from build123d import *

# Parameters (mm, degrees)
EXTRUDE_1_DEPTH     = 20
EXTRUDE_2_DEPTH     = 20
SKETCH_11_W         = 6.4
SKETCH_11_H         = 6.4
CUT_EXTRUDE_2_DEPTH = 13.1
SKETCH_4_R          = 1.6
CUT_EXTRUDE_1_DEPTH = 9.2


with BuildPart() as part:
    # 草图3 → 凸台-拉伸1 (new body)
    with BuildSketch(Plane.XY):
        Polygon((0, 0), (20, -12.790533612), (20, -72.995577455), (0, -72.995577455), align=None)
    extrude(amount=EXTRUDE_1_DEPTH)

    # 草图6 → 凸台-拉伸2 (add)
    with BuildSketch(Plane.XY.offset(20)):
        Polygon((0, -72.995577455), (-15, -72.995577455), (-15, -69.995577455), (0, 0), (0, -69.995577455), align=None)
    extrude(amount=-EXTRUDE_2_DEPTH)

    # 草图11 → 切除-拉伸2 (cut)
    with BuildSketch(Plane.XY.offset(20)):
        with Locations((-7.5, -66.995577455)):
            Rectangle(SKETCH_11_W, SKETCH_11_H)
        with Locations((10, -66.995577455)):
            Rectangle(SKETCH_11_W, SKETCH_11_H)
    extrude(amount=-CUT_EXTRUDE_2_DEPTH, mode=Mode.SUBTRACT)

    # 草图4 → 切除-拉伸1 (cut)
    with BuildSketch(Plane.XZ.offset(72.995577455)):
        with Locations(Location((10, 10, 0), (0, 0, 270))):
            Circle(SKETCH_4_R)
        with Locations(Location((-7.5, 10, 0), (0, 0, 270))):
            Circle(SKETCH_4_R)
    extrude(amount=-CUT_EXTRUDE_1_DEPTH, mode=Mode.SUBTRACT)


solid = part.part
Here's how the part is built. I have some questions about the finished solid (model axes, mm). A direction names the side the tool comes from. Give positions to 0.01 mm unless a question says otherwise; leave off trailing zeros. Loops run counter-clockwise (first coordinate to the right, second up) from the corner with the lowest first, then second, coordinate; pieces in that order, holes last. Notation, with made-up numbers: (88.5, -28.5) -> (96.5, -28.5) arc R20 ccw to (96.5, -8.5) -> close; hole circle Ø5 at (-17.5, -14.75). An arc over 180 degrees is marked (long way). Answer as a JSON object with one key per item and string values. Group by question number.
Item 1: Imagine slicing it at C-C on z = 10. Write out the boundary of the cut face in (x, y), then the cut area to 3 significant figures.
Item 2: I need wall thicknesses on L1, parallel to X at y = -71, z = 10; L2, parallel to Y at x = 9, z = 12.75; L3, parallel to Y at x = 7.5, z = 11.5. Which ranges of each line are inside material? Lowest first, please.
Item 3: On a 3-axis mill with a long thin cutter (end or side, diameter ignored), from which of +Z, -Z, +X, -X, +Y, -Y can I reach the whole of each face in a straight line? I mean faces 4 (the cylindrical face through (-8.47, -71.62, 11.27)), 5 (the flat face through (-4.3, -67, 14)), 6 (the flat face through (7, -44, 20)). Say none if no direction works.
Item 4: Will these pins go through, and if not, where does the flat tip stop? pin 1 (7 mm diameter, centred on x = 9.5, z = 11.5, fed in from +Y); pin 2 (1.9 mm diameter, centred on y = -65.5, z = 14, fed in from -X); pin 3 (3.5 mm diameter, centred on x = 10, z = 10, fed in from +Y).
Item 5: Thinking about a two-plate mould opening in Y: for faces 1 (the flat face through (3, -72.996, 10)), 2 (the flat face through (6.8, -67, 14)), 3 (the flat face through (-15, -72, 10)), which applies, pulls with the +Y half, pulls with the -Y half, needs draft (parallel to the pull), parting line crosses it, or undercut?
Item 6: Imagine slicing it at B-B on x = 10. Write out the boundary of the cut face in (y, z).
Item 7: Imagine slicing it at A-A on z = 15.25. Write out the boundary of the cut face in (x, y).
Item 8: Imagine slicing it at D-D on x = -7.5. Write out the boundary of the cut face in (y, z).
Answer list:
{
 "1": {"outline": "(-15, -73) -> (-9.1, -73) -> (-9.1, -70.2) -> (-10.7, -70.2) -> (-10.7, -63.8) -> (-4.3, -63.8) -> (-4.3, -70.2) -> (-5.9, -70.2) -> (-5.9, -73) -> (8.4, -73) -> (8.4, -70.2) -> (6.8, -70.2) -> (6.8, -63.8) -> (13.2, -63.8) -> (13.2, -70.2) -> (11.6, -70.2) -> (11.6, -73) -> (20, -73) -> (20, -12.79) -> (0, 0) -> (-15, -70) -> close", "area": "1,800 mm2"},
 "2": {"L1": "x = -15 to -9.1, -5.9 to 8.4, 11.6 to 20", "L2": "y = -73 to -70.2, -63.8 to -5.76", "L3": "y = -73 to -70.2, -63.8 to -4.8"},
 "3": {"face 4": "-Y", "face 5": "+Z", "face 6": "+Z, +X, -X, +Y, -Y"},
 "4": {"pin 1": "stops at y = -3.84", "pin 2": "stops at x = -14.24", "pin 3": "stops at y = -5.28"},
 "5": {"face 1": "pulls with the -Y half", "face 2": "undercut", "face 3": "needs draft"},
 "6": {"outline": "(-73, 0) -> (-6.4, 0) -> (-6.4, 20) -> (-63.8, 20) -> (-63.8, 6.9) -> (-70.2, 6.9) -> (-70.2, 8.4) -> (-73, 8.4) -> close; (-73, 11.6) -> (-70.2, 11.6) -> (-70.2, 20) -> (-73, 20) -> close"},
 "7": {"outline": "(-15, -73) -> (20, -73) -> (20, -12.79) -> (0, 0) -> (-15, -70) -> close; hole (-10.7, -70.2) -> (-4.3, -70.2) -> (-4.3, -63.8) -> (-10.7, -63.8) -> close; hole (6.8, -70.2) -> (13.2, -70.2) -> (13.2, -63.8) -> (6.8, -63.8) -> close"},
 "8": {"outline": "(-73, 0) -> (-35, 0) -> (-35, 20) -> (-63.8, 20) -> (-63.8, 6.9) -> (-70.2, 6.9) -> (-70.2, 8.4) -> (-73, 8.4) -> close; (-73, 11.6) -> (-70.2, 11.6) -> (-70.2, 20) -> (-73, 20) -> close"}
}
